Input: part model. Units: mm. Frame: model coordinates. Face numbers are marked on the shaded views. A direction names the side the tool comes from. Round coordinates to 2 decimals unless told otherwise and drop trailing zeros. Order: outer loops, then holes, each group sorted by start corner. A loop starts at its lowest first (then second) coordinate and runs counter-clockwise, first axis right, second up.
Item 1: Cut plane A-A on z = 10. Give the number of separate pieces and of enclosed holes in the cut face, then the cut area to 3 significant figures.
Item 2: Mould query, pull axis X, two halves, no side actions, for the marked faces 1, 2 and 3. Classes: released by +X, released by -X, zero draft, split by the parting line, or undercut.
Item 3: Line query: L1, parallel to Z at x = 7.5, y = 2.2; L2, parallel to Y at x = 98, z = 2.75; L3, parallel to X at y = 8, z = 8.5. Output: solid intervals per line, ascending.
Item 4: Cut plane B-B on x = 68. Output: boundary loops of the cut face in (y, z), then the cut area to 3 significant figures.
Item 5: First-contact query: pin 1 (10 mm diameter, centred on y = 31, z = 12, fed in from -X); pin 2 (3 mm diameter, centred on x = 5.5, z = 17.5, fed in from -Y); pin 3 (4 mm diameter, centred on x = 77.5, y = 25, fed in from +Z). Flat tips, straight axial feed; report the tip coordinate or a pass-through.
Item 6: Reachability of the marked faces 4 and 5 from +Z, -Z, +X, -X, +Y, -Y: full face, straight path, thin tool, end or side. Return the list, or none.
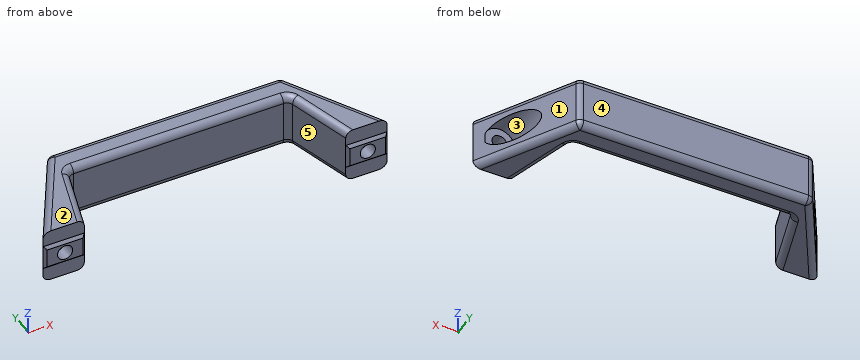
```python
from build123d import *

# Parameters (mm, degrees)
F1_DEPTH = 20
F2_W     = 15
F2_H     = 9
F3_DEPTH = 1
F4_R     = 2.75
F5_DEPTH = 36.001
F6_R     = 5.5
F7_DEPTH = 31
F8_F1_R  = 2.5
F8_F2_R  = 2.5
F9_SIZE  = 0.99999


# Not quite as in the source:
# - a fillet or chamfer is up to 0.001 mm smaller than in the source, because OpenCascade refuses the exact size


with BuildPart() as f1:
    # F0 (on Top) → F1 (new body)
    with BuildSketch(Plane.XY):
        Polygon((20.2072594216, 35), (0, 0), (15, 0), (22.5, 25), (102.5, 25), (110, 0), (125, 0), (104.7927405784, 35), align=None)
    extrude(amount=F1_DEPTH)

    # F2 (on face) → F3 (join)
    with BuildSketch(Plane.XZ):
        with Locations((7.5, 10)):
            Rectangle(F2_W, F2_H)
        with Locations((117.5, 10)):
            Rectangle(F2_W, F2_H)
    extrude(amount=F3_DEPTH)

    # F4 (on face) → F5 (cut, through all)
    with BuildSketch(Plane.XZ.offset(1)):
        with Locations((7.5, 10)):
            Circle(F4_R)
        with Locations((117.5, 10)):
            Circle(F4_R)
    extrude(amount=-F5_DEPTH, mode=Mode.SUBTRACT)

    # F6 (on face) → F7 (cut)
    with BuildSketch(Plane(origin=(0, 35, 0), x_dir=(-1, 0, 0), z_dir=(0, 1, 0))):
        with Locations((-117.5, 10)):
            Circle(F6_R)
        with Locations((-7.5, 10)):
            Circle(F6_R)
    extrude(amount=-F7_DEPTH, mode=Mode.SUBTRACT)

    # F8: fillet of radius 2.5 on 12 edges, made by hand

    # F8_f1
    f8_f1_edges = [f1.edges().sort_by_distance(p)[0] for p in [
        (22.5, 25, 10),
        (102.5, 25, 10),
    ]]
    fillet(f8_f1_edges, radius=F8_F1_R)

    # F8_f2
    f8_f2_edges = [f1.edges().sort_by_distance(p)[0] for p in [
        (62.5, 25, 0),
        (62.5, 25, 20),
        (104.7927405784, 35, 10),
        (20.2072594216, 35, 10),
        (62.5, 35, 0),
        (62.5, 35, 20),
        (114.8963702892, 17.5, 20),
        (114.8963702892, 17.5, 0),
        (10.1036297108, 17.5, 20),
        (10.1036297108, 17.5, 0),
        (22.8677503031, 24.5057323207, 20),
        (102.1322496969, 24.5057323207, 20),
        (22.8677503031, 24.5057323207, 0),
        (102.1322496969, 24.5057323207, 0),
    ]]
    fillet(f8_f2_edges, radius=F8_F2_R)

    # F9 (size 1 in the source; OpenCascade refuses exactly that, so slightly less here)
    f9_edges = [f1.edges().sort_by_distance(p)[0] for p in [
        (7.5, -1, 14.5),
        (0, -1, 10),
        (7.5, -1, 5.5),
        (15, -1, 10),
        (117.5, -1, 14.5),
        (110, -1, 10),
        (117.5, -1, 5.5),
        (125, -1, 10),
    ]]
    chamfer(f9_edges, length=F9_SIZE)


solid = f1.part
```
From the geometry:
1. separate pieces: 3
1. enclosed holes: 0
1. area: 1,260 mm2
2. face 1: released by +X
2. face 2: zero draft
2. face 3: undercut
3. L1: z = 0 to 7.25, 12.75 to 20
3. L2: y = 25 to 35
3. L3: x = 12.79 to 17.4, 107.6 to 112.21
4. outline: (25, 2.5) arc R2.5 ccw to (27.5, 0) - (32.5, 0) arc R2.5 ccw to (35, 2.5) - (35, 17.5) arc R2.5 ccw to (32.5, 20) - (27.5, 20) arc R2.5 ccw to (25, 17.5) - close
4. area: 195 mm2
5. pin 1: stops at x = 15.01
5. pin 2: stops at y = 0
5. pin 3: stops at z = 19.95
6. face 4: +Z, -Z, +X, -X, +Y
6. face 5: +Z, -Z, -Y
